Here's the drawing with two shaded views (mm, measured from the low corner). I have some questions. A direction names the side the tool comes from. Round coordinates to 2 decimals unless told otherwise and drop trailing zeros. Order: outer loops, then holes, each group sorted by start corner. A loop starts at its lowest first (then second) coordinate and runs counter-clockwise, first axis right, second up.
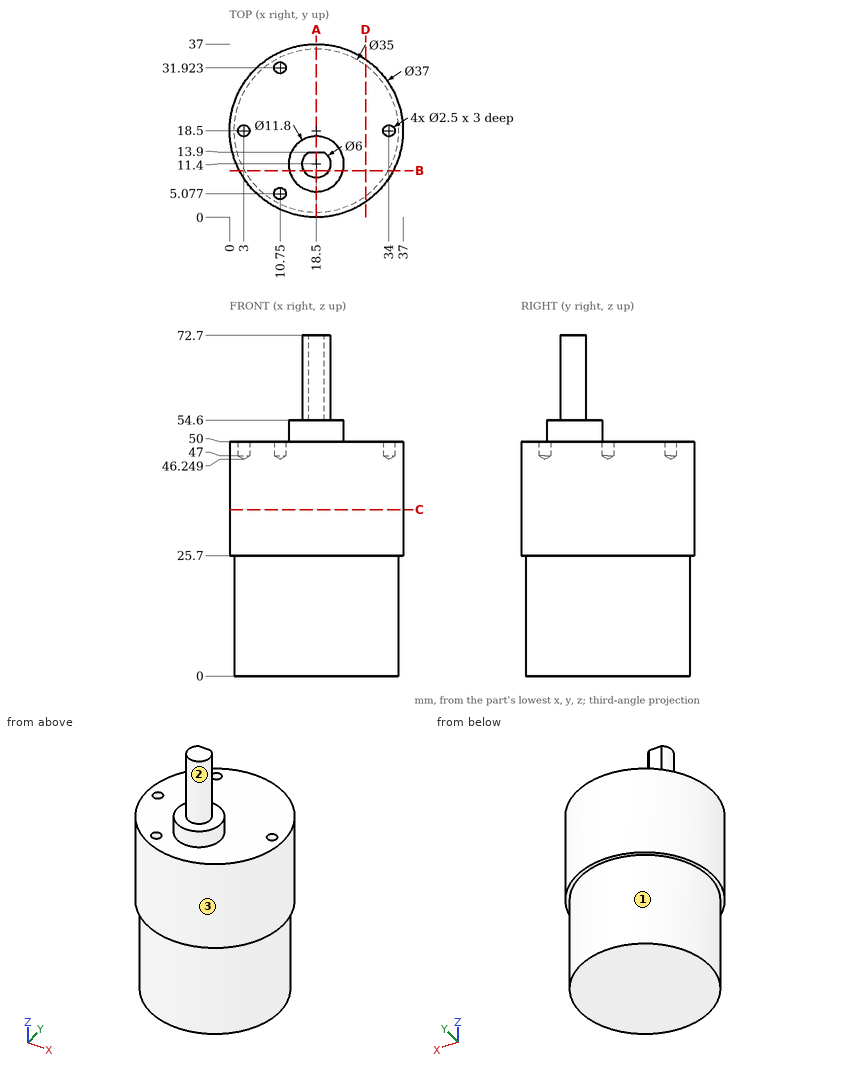
Q1. I need wall thicknesses on L1, parallel to X at y = 18.5, z = 48.5; L2, parallel to X at y = 18, z = 48 (1 decimal); L3, parallel to Z at x = 16, y = 13.5. Which ranges of each line are inside material? Lowest first, please.
Q2. Imagine slicing it at D-D, the plane x = 29. Please give me the cut outline in (y, z), then the cut area to 3 significant figures.
Q3. Imagine slicing it at C-C, the plane z = 35.5. Please give me the cut outline in (x, y).
Q4. For P1, Ø2, axis at x = 3, y = 18.5, coming from the +Z side; P2, Ø1, axis at x = 4.5, y = 31.5, coming from the -Z side; P3, Ø8, axis at x = 32, z = 41, coming from the -Y side (1 decimal); P4, Ø1.5, axis at x = 34, y = 18.5, coming from the +Z side, each with a flat end and sliding along its axis, tell me the tip position at first contact or that it passes through.
Q5. For the marked faces 1, 2 and 3, which set-ups out of +Z, -Z, +X, -X, +Y, -Y let a thin tool reach every point of the face, with its end or its side?
Q6. Imagine slicing it at B-B, the plane y = 10. Please give me the cut outline in (x, z), then the cut area to 3 significant figures.
Q7. Imagine slicing it at A-A, the plane x = 18.5. Please give me the cut outline in (y, z).
Filled in:
1. L1: x = 0 to 1.75, 4.25 to 32.75, 35.25 to 37
1. L2: x = 0 to 1.9, 4.1 to 32.9, 35.1 to 37
1. L3: z = 0 to 54.6
2. outline: (3.27, 25.7) - (4.5, 25.7) - (4.5, 0) - (32.5, 0) - (32.5, 25.7) - (33.73, 25.7) - (33.73, 50) - (3.27, 50) - close
2. area: 1,460 mm2
3. outline: circle Ø37 at (18.5, 18.5)
4. P1: stops at z = 46.85
4. P2: passes through
4. P3: stops at y = 2.6
4. P4: stops at z = 46.7
5. face 1: -Z
5. face 2: +Z
5. face 3: +Z, -Z
6. outline: (2.07, 25.7) - (3.2, 25.7) - (3.2, 0) - (33.8, 0) - (33.8, 25.7) - (34.93, 25.7) - (34.93, 50) - (24.23, 50) - (24.23, 54.6) - (21.15, 54.6) - (21.15, 72.7) - (15.85, 72.7) - (15.85, 54.6) - (12.77, 54.6) - (12.77, 50) - (2.07, 50) - close
6. area: 1,730 mm2
7. outline: (0, 25.7) - (1, 25.7) - (1, 0) - (36, 0) - (36, 25.7) - (37, 25.7) - (37, 50) - (17.3, 50) - (17.3, 54.6) - (13.9, 54.6) - (13.9, 72.7) - (8.4, 72.7) - (8.4, 54.6) - (5.5, 54.6) - (5.5, 50) - (0, 50) - close
